Design review of the part built by this model. Coordinates are the model's own, in mm. Coordinates: 2 decimals unless noted, no trailing zeros. Order: outer loops, then holes, each group sorted by start corner. A loop starts at its lowest first (then second) coordinate and runs counter-clockwise, first axis right, second up. Notation, with made-up numbers: M 81,-6 L 134,-6 A17 cw 134,7 Z; hole C -7,85.25 d5. An arc over 180 degrees is marked long. Answer in a Markdown table with one row per item.
from build123d import *

# Parameters (mm, degrees)
SKETCH1_R      = 5.75
SKETCH1_R_2    = 41.75
EXTRUDE1_DEPTH = 0.5


with BuildPart() as part:
    # Sketch1 → Extrude1 (new body)
    with BuildSketch(Plane.XY):
        with BuildLine():
            Line((-40.75, 50.75), (40.75, 50.75))
            ThreePointArc((40.75, 50.75), (47.821067812, 47.821067812), (50.75, 40.75))
            Line((50.75, 40.75), (50.75, -40.75))
            ThreePointArc((50.75, -40.75), (47.821067812, -47.821067812), (40.75, -50.75))
            Line((40.75, -50.75), (-40.75, -50.75))
            ThreePointArc((-40.75, -50.75), (-47.821067812, -47.821067812), (-50.75, -40.75))
            Line((-50.75, -40.75), (-50.75, 40.75))
            ThreePointArc((-50.75, 40.75), (-47.821067812, 47.821067812), (-40.75, 50.75))
        make_face()
        with Locations((37.618080759, 37.618080759)):
            Circle(SKETCH1_R, mode=Mode.SUBTRACT)
        with Locations(Location((-37.618080759, 37.618080759, 0), (0, 0, 180))):
            Circle(SKETCH1_R, mode=Mode.SUBTRACT)
        with Locations((-37.618080759, -37.618080759)):
            Circle(SKETCH1_R, mode=Mode.SUBTRACT)
        with Locations(Location((37.618080759, -37.618080759, 0), (0, 0, 180))):
            Circle(SKETCH1_R, mode=Mode.SUBTRACT)
        Circle(SKETCH1_R_2, mode=Mode.SUBTRACT)
    extrude(amount=EXTRUDE1_DEPTH)


solid = part.part
(1) Add section A-A, the plane x = 0. Give the boundary of the cut face in (y, z), and give its area (3 significant figures).
Return value:
| item | result |
|---|---|
| outline | M -50.75,0 L -41.75,0 L -41.75,0.5 L -50.75,0.5 Z; M 41.75,0 L 50.75,0 L 50.75,0.5 L 41.75,0.5 Z |
| area | 9.00 mm2 |
(2) Draft analysis for pull direction Y (two halves, no side actions). For faces 1 (the flat face through (-44, 1, 0.5)), 2 (the cylindrical face through (47.74, 47.9, 0.25)), 3 (the cylindrical face through (-36.37, 43.23, 0.25)), state which applies: pulls with the +Y half, pulls with the -Y half, needs draft (parallel to the pull), parting line crosses it, or undercut.
Return value:
| item | result |
|---|---|
| face 1 | needs draft |
| face 2 | pulls with the +Y half |
| face 3 | undercut |
(3) Add section C-C, the plane z = 0.1. Give the boundary of the cut face in (x, y), and give its area (3 significant figures).
Return value:
| item | result |
|---|---|
| outline | M -50.75,-40.75 A10 ccw -40.75,-50.75 L 40.75,-50.75 A10 ccw 50.75,-40.75 L 50.75,40.75 A10 ccw 40.75,50.75 L -40.75,50.75 A10 ccw -50.75,40.75 Z; hole C -37.62,-37.62 d11.5; hole C -37.62,37.62 d11.5; hole C 0,0 d83.5; hole C 37.62,-37.62 d11.5; hole C 37.62,37.62 d11.5 |
| area | 4,320 mm2 |
(4) For line 1 along X through (y, z) = (-9, 0.3); line 2 along Y through (x, z) = (0.5, 0.45); line 3 along Y through (x, z) = (27, 0.2), list the stretches that pass through material, from the lowest coordinate up. Write a range as from..to.
Return value:
| item | result |
|---|---|
| line 1 | x = -50.75..-40.77, 40.77..50.75 |
| line 2 | y = -50.75..-41.75, 41.75..50.75 |
| line 3 | y = -50.75..-31.84, 31.84..50.75 |
